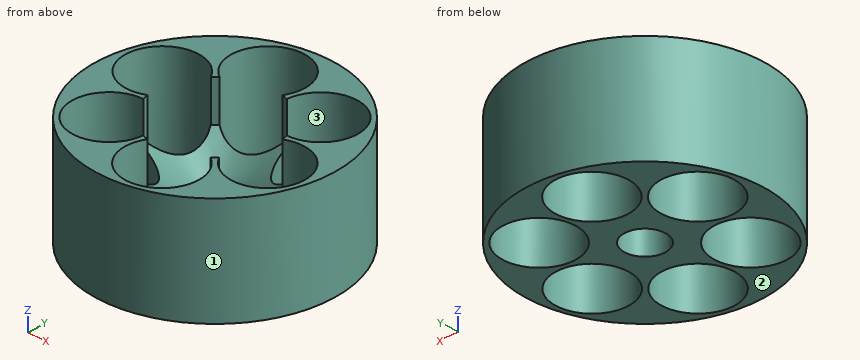
```python
from build123d import *

# Parameters (mm, degrees)
F0_R     = 18.375
F1_DEPTH = 16.45
F3_D     = 11.3
F5_D     = 18.25
F5_DEPTH = 6.3
F5_TIP   = 5.4828531486
F7_D     = 6.35


with BuildPart() as f1:
    # F0 (on Top) → F1 (new body)
    with BuildSketch(Plane.XY):
        Circle(F0_R)
    extrude(amount=F1_DEPTH)

    # F3 (through all)
    with Locations(Plane.XY.offset(16.45)):
        with Locations((-8.8218893741, -8.1347567801), (-2.6339613381, 11.7073586974), (-11.4558507122, 3.5726019173), (2.6339613381, -11.7073586974), (11.4558507122, -3.5726019173), (8.8218893741, 8.1347567801)):
            Hole(F3_D / 2)

    # F5
    with Locations(Plane.XY.offset(16.45)):
        with Locations((0, 0)):
            Hole(F5_D / 2, depth=F5_DEPTH)
            with Locations((0, 0, -(F5_DEPTH + F5_TIP / 2))):  # 118° drill point
                Cone(0, F5_D / 2, F5_TIP, mode=Mode.SUBTRACT)

    # F7 (through all)
    with Locations(Plane(origin=(0, 0, 0), x_dir=(1, 0, 0), z_dir=(0, 0, -1))):
        with Locations((0, 0)):
            Hole(F7_D / 2)


solid = f1.part
```
Source: CAD feature listing. Evaluate the final solid. Frame: model axes, mm. Face numbers are marked on the shaded views. Round coordinates to 2 decimals unless told otherwise and drop trailing zeros. Loops run counter-clockwise (first coordinate to the right, second up) from the corner with the lowest first, then second, coordinate; pieces in that order, holes last. Notation, with made-up numbers: M 31,60.25 L 55,60.25 A28 ccw 55,91.25 Z; hole C -31.75,-10 d2. An arc over 180 degrees is marked long. Use a Markdown table: item, result. Add a question column.
1. Section query A-A on y = 0. Return the cut outline in (x, z) (3 decimals).
2. Section query C-C on z = 2. Return the cut outline in (x, y) (3 decimals), then the cut area to 3 significant figures.
3. Contact query for flat-ended pins moving along their axis: P1, Ø8, axis at y = -7.5, z = 9, coming from the +X side; P2, Ø4, axis at x = 5, y = 1.5, coming from the +Z side; P3, Ø14.5, axis at x = -11.46, y = 3.57, coming from the -Z side; P4, Ø5, axis at x = 3.5, y = -5, coming from the +Z side. Output: stop coordinate, or through.
4. Section query B-B on x = -12. Return the cut outline in (y, z), then the cut area to 3 significant figures.
5. Mould query, pull axis Y, two halves, no side actions, for the marked faces 1, 2 and 3. Classes: pulls with the +Y half, pulls with the -Y half, needs draft (parallel to the pull), parting line crosses it, or undercut.
6. Section query D-D on x = 0. Return the cut outline in (y, z) (3 decimals).
7. Line query: line 1 (X direction, y = -3.5, z = 4.25); line 2 (Y direction, x = -7, z = 13.5); line 3 (Y direction, x = 11, z = 5.5). Output: solid intervals per line, ascending.
Reported:
| question | item | result |
|---|---|---|
| 1 | outline | M -18.375,0 L -15.833,0 L -15.833,16.45 L -18.375,16.45 Z; M -7.079,0 L -3.175,0 L -3.175,6.575 L -7.079,8.92 Z; M 3.175,0 L 7.079,0 L 7.079,8.92 L 3.175,6.575 Z; M 15.833,0 L 18.375,0 L 18.375,16.45 L 15.833,16.45 Z |
| 2 | outline | C 0,0 d36.75; hole C -11.456,3.573 d11.3; hole C -8.822,-8.135 d11.3; hole C -2.634,11.707 d11.3; hole C 0,0 d6.35; hole C 2.634,-11.707 d11.3; hole C 8.822,8.135 d11.3; hole C 11.456,-3.573 d11.3 |
| 2 | area | 427 mm² |
| 3 | P1 | stops at x = 18.04 |
| 3 | P2 | stops at z = 9.01 |
| 3 | P3 | stops at z = 0 |
| 3 | P4 | stops at z = 9.82 |
| 4 | outline | M -13.92,0 L -12.81,0 L -12.81,16.45 L -13.92,16.45 Z; M -3.46,0 L -2.05,0 L -2.05,16.45 L -3.46,16.45 Z; M 9.2,0 L 13.92,0 L 13.92,16.45 L 9.2,16.45 Z |
| 4 | area | 119 mm² |
| 5 | face 1 | parting line crosses it |
| 5 | face 2 | needs draft |
| 5 | face 3 | undercut |
| 6 | outline | M -18.375,0 L -16.706,0 L -16.706,16.45 L -18.375,16.45 Z; M -6.709,0 L -3.175,0 L -3.175,6.575 L -6.709,8.698 Z; M 3.175,0 L 6.709,0 L 6.709,8.698 L 3.175,6.575 Z; M 16.706,0 L 18.375,0 L 18.375,16.45 L 16.706,16.45 Z |
| 7 | line 1 | x = -18.04 to -12.05, -5.59 to 5.81, 17.11 to 18.04 |
| 7 | line 2 | y = -16.99 to -13.48, 7.05 to 8.12, 15.29 to 16.99 |
| 7 | line 3 | y = -14.72 to -9.2, 2.06 to 2.92, 13.35 to 14.72 |
